from build123d import *

# Parameters (mm, degrees)
F1_DEPTH = 45.5
F2_W     = 61.5
F2_H     = 61
F3_DEPTH = 21.001
F4_W     = 3.5
F4_H     = 51
F5_DEPTH = 21.001
F6_W     = 87.66
F6_H     = 1.44
F7_DEPTH = 6


# Not quite as in the source:
# - a pattern or mirror of a feature is missing from the dataset's text; its kind, count and spacing are read off the source's solid


with BuildPart() as f1:
    # F0 (on Front) → F1 (new body, symmetric)
    with BuildSketch(Plane.XZ):
        Polygon((45.75, 21), (-45.75, 21), (-45.75, 8.5), (-49.25, 5), (-45.75, 1.5), (-45.75, 0), (-43.83, 0), (-43.83, 19), (43.83, 19), (43.83, 0), (45.75, 0), (45.75, 1.5), (49.25, 5), (45.75, 8.5), align=None)
    extrude(amount=F1_DEPTH, both=True)

    # F2 (on face) → F3 (cut, through all)
    with BuildSketch(Plane.XY.offset(21)):
        Rectangle(F2_W, F2_H)
    extrude(amount=-F3_DEPTH, mode=Mode.SUBTRACT)

    # F4 (on face) → F5 (cut, through all)
    with BuildSketch(Plane.XY.offset(21)):
        with Locations((47.5, 0)):
            Rectangle(F4_W, F4_H)
    f5 = extrude(amount=-F5_DEPTH, mode=Mode.SUBTRACT)

    # F5_copies: F5 across plane
    add(f5.mirror(Plane(origin=(0, 0, 0), x_dir=(0, 0, -1), z_dir=(-1, 0, 0))), mode=Mode.SUBTRACT)

    # F6 (on face) → F7 (join)
    with BuildSketch(Plane(origin=(0, 0, 19), x_dir=(1, 0, 0), z_dir=(0, 0, -1))):
        with Locations((0, 44.78)):
            Rectangle(F6_W, F6_H)
    f7 = extrude(amount=F7_DEPTH)

    # F7_copies: F7 across plane
    add(f7.mirror(Plane.ZX))


solid = f1.part
Input: part model. Units: mm. Frame: model coordinates. A direction names the side the tool comes from. Coordinates: 2 decimals unless noted, no trailing zeros. Loops run counter-clockwise (first coordinate to the right, second up) from the corner with the lowest first, then second, coordinate; pieces in that order, holes last. Notation, with made-up numbers: (8, 3) - (15, 3) arc R15 cw to (15, 31) - close; hole circle Ø8 at (38.25, 43). An arc over 180 degrees is marked (long way). Answer in a Markdown table with one row per item. Add a question column.
Item 1: Access query for faces 1 (the flat face through (47, -25.5, 5)), 2 (the flat face through (-47, -25.5, 5)), 3 (the flat face through (43.83, -1, 10)). Directions: +Z, -Z, +X, -X, +Y, -Y. A direction counts if a zero-diameter tool reaches every point of the face in a straight line with its end or side. Return the directions, or none.
Item 2: Section query C-C on x = -23. Return the cut outline in (y, z), then the cut area to 3 significant figures.
Item 3: Section query A-A on y = 5.5. Return the cut outline in (x, z), then the cut area to 3 significant figures.
Item 4: Mould query, pull axis X, two halves, no side actions, for faces 4 (the flat face through (-47, 25.5, 5)), 5 (the flat face through (47.48, -35.64, 3.23)), 6 (the flat face through (-1, 44.06, 16)). Classes: released by +X, released by -X, zero draft, split by the parting line, or undercut.
Item 5: Line query: line 1 along X through (y, z) = (25, 18); line 2 along Y through (x, z) = (-14, 17.5); line 3 along X through (y, z) = (-37.5, 5). Output: solid intervals per line, ascending. Write a range as [from, to].
Item 6: Section query D-D on y = 34. Return the cut outline in (x, z).
Item 7: Section query B-B on z = 3. Return the cut outline in (x, y).
Item 8: Contact query for flat-ended pins moving along their axis: P1, Ø1.6, axis at y = -12, z = 20.5, coming from the +X side; P2, Ø1.6, axis at x = 18, y = -45, coming from the -Z side; P3, Ø1, axis at y = 13, z = 19.5, coming from the -X side. Output: stop coordinate, or through.
Recorded:
| question | item | result |
|---|---|---|
| 1 | face 1 | +Z, -Z, +X |
| 1 | face 2 | +Z, -Z, -X |
| 1 | face 3 | -Z |
| 2 | outline | (-45.5, 13) - (-44.06, 13) - (-44.06, 19) - (-30.5, 19) - (-30.5, 21) - (-45.5, 21) - close; (30.5, 19) - (44.06, 19) - (44.06, 13) - (45.5, 13) - (45.5, 21) - (30.5, 21) - close |
| 2 | area | 77.3 mm^2 |
| 3 | outline | (-45.75, 0) - (-43.83, 0) - (-43.83, 19) - (-30.75, 19) - (-30.75, 21) - (-45.75, 21) - close; (30.75, 19) - (43.83, 19) - (43.83, 0) - (45.75, 0) - (45.75, 21) - (30.75, 21) - close |
| 3 | area | 133 mm^2 |
| 4 | face 4 | zero draft |
| 4 | face 5 | released by +X |
| 4 | face 6 | undercut |
| 5 | line 1 | [-45.75, -43.83], [43.83, 45.75] |
| 5 | line 2 | [-45.5, -44.06], [44.06, 45.5] |
| 5 | line 3 | [-49.25, -43.83], [43.83, 49.25] |
| 6 | outline | (-49.25, 5) - (-45.75, 1.5) - (-45.75, 0) - (-43.83, 0) - (-43.83, 19) - (43.83, 19) - (43.83, 0) - (45.75, 0) - (45.75, 1.5) - (49.25, 5) - (45.75, 8.5) - (45.75, 21) - (-45.75, 21) - (-45.75, 8.5) - close |
| 7 | outline | (-47.25, -45.5) - (-43.83, -45.5) - (-43.83, 45.5) - (-47.25, 45.5) - (-47.25, 25.5) - (-45.75, 25.5) - (-45.75, -25.5) - (-47.25, -25.5) - close; (43.83, -45.5) - (47.25, -45.5) - (47.25, -25.5) - (45.75, -25.5) - (45.75, 25.5) - (47.25, 25.5) - (47.25, 45.5) - (43.83, 45.5) - close |
| 8 | P1 | x = 45.75 |
| 8 | P2 | z = 13 |
| 8 | P3 | x = -45.75 |
